from build123d import *

# Parameters (mm, degrees)
REVOLVE1_ANGLE           = 180
SKETCH3_R                = 2
BOSS_EXTRUDE1_DEPTH      = 13
BOSS_EXTRUDE8_REACH      = 185.507
BOSS_EXTRUDE8_END_RADIUS = 88.5
SKETCH7_R                = 10
SKETCH7_R_2              = 1.5
CUT_EXTRUDE1_DEPTH       = 10
BOSS_EXTRUDE11_DEPTH     = 25
FILLET1_R                = 20
CUT_EXTRUDE2_DEPTH       = 10
CUT_EXTRUDE3_DEPTH       = 10


with BuildPart() as part:
    # Sketch1 → Revolve1 (revolve)
    with BuildSketch(Plane(origin=(0, 0, 0), x_dir=(1, 0, 0), z_dir=(0, 1, 0))):
        Polygon((0, 75), (95, 75), (95, -95), (0, -125), align=None)
    revolve(axis=Axis((0, 0, 125), (0, 0, -1)), revolution_arc=REVOLVE1_ANGLE)

    # Sketch2 → Cut-Revolve3 (revolve, cut)
    with BuildSketch(Plane(origin=(0, 0, 0), x_dir=(1, 0, 0), z_dir=(0, 1, 0))):
        Polygon((0, 68.5), (0, -118.183600921), (88.5, -90.2362325), (88.5, 68.5), align=None)
    revolve(axis=Axis((0, 0, -68.5), (0, 0, 1)), mode=Mode.SUBTRACT)

    # Sketch3 → Boss-Extrude1 (add)
    with BuildSketch(Plane(origin=(0, 0, 0), x_dir=(1, 0, 0), z_dir=(0, 1, 0))):
        with Locations((-91.75, 56.5)):
            Circle(SKETCH3_R)
        with Locations((-91.75, 26.5)):
            Circle(SKETCH3_R)
        with Locations((-91.75, -18.5)):
            Circle(SKETCH3_R)
        with Locations((-91.75, -54.5)):
            Circle(SKETCH3_R)
        with Locations((91.75, -54.5)):
            Circle(SKETCH3_R)
        with Locations((91.75, -18.5)):
            Circle(SKETCH3_R)
        with Locations((91.75, 26.5)):
            Circle(SKETCH3_R)
        with Locations((91.75, 56.5)):
            Circle(SKETCH3_R)
    extrude(amount=BOSS_EXTRUDE1_DEPTH)

    # Boss-Extrude8: up to this cylinder (the profile starts inside it)
    boss_extrude8_end = Plane(origin=(0, 0, -64.648778), z_dir=(0, 0, -1)) * Cylinder(BOSS_EXTRUDE8_END_RADIUS, 549.014, mode=Mode.PRIVATE)
    # Sketch5 → Boss-Extrude8 (add, up to the surface)
    with BuildSketch(Plane(origin=(0, 0, 0), x_dir=(1, 0, 0), z_dir=(0, 1, 0)), mode=Mode.PRIVATE) as boss_extrude8_sk1:
        with BuildLine():
            Line((23.5, 63.447630747), (23.5, 68.5))
            Line((23.5, 68.5), (26.5, 68.5))
            Line((26.5, 68.5), (26.5, 63.447630747))
            Line((26.5, 63.447630747), (27.4, 63.447630747))
            ThreePointArc((27.4, 63.447630747), (25, 61.047630747), (22.6, 63.447630747))
            Line((22.6, 63.447630747), (23.5, 63.447630747))
        make_face()
    boss_extrude8_tool1 = extrude(boss_extrude8_sk1.sketch, amount=-BOSS_EXTRUDE8_REACH, mode=Mode.PRIVATE) & boss_extrude8_end
    add(boss_extrude8_tool1.solids().sort_by_distance((25, 0, -64.648778))[0])
    # Sketch5 → Boss-Extrude8 (add, up to the surface)
    with BuildSketch(Plane(origin=(0, 0, 0), x_dir=(1, 0, 0), z_dir=(0, 1, 0)), mode=Mode.PRIVATE) as boss_extrude8_sk2:
        with BuildLine():
            Line((-27.4, 63.447630747), (-26.5, 63.447630747))
            Line((-26.5, 63.447630747), (-26.5, 68.5))
            Line((-26.5, 68.5), (-23.5, 68.5))
            Line((-23.5, 68.5), (-23.5, 63.447630747))
            Line((-23.5, 63.447630747), (-22.6, 63.447630747))
            ThreePointArc((-22.6, 63.447630747), (-25, 61.047630747), (-27.4, 63.447630747))
        make_face()
    boss_extrude8_tool2 = extrude(boss_extrude8_sk2.sketch, amount=-BOSS_EXTRUDE8_REACH, mode=Mode.PRIVATE) & boss_extrude8_end
    add(boss_extrude8_tool2.solids().sort_by_distance((-25, 0, -64.648778))[0])

    # Sketch7 → Cut-Extrude1 (cut)
    with BuildSketch(Plane.XY.offset(-68.5)):
        Circle(SKETCH7_R)
        with Locations((20.425168298, -1.75)):
            Circle(SKETCH7_R_2)
        with Locations(Location((-20.425168298, -1.75, 0), (0, 0, 180))):
            Circle(SKETCH7_R_2)
    extrude(amount=-CUT_EXTRUDE1_DEPTH, mode=Mode.SUBTRACT)

    # Sketch8 → Boss-Extrude11 (add, symmetric)
    with BuildSketch(Plane.XY):
        Polygon((90.138781887, -30), (130.138781887, -30), (92.29707471, -22.5), align=None)
        Polygon((-130.138781887, -30), (-92.29707471, -22.5), (-90.138781887, -30), align=None)
    extrude(amount=BOSS_EXTRUDE11_DEPTH, both=True)

    # Fillet1
    fillet1_edges = [part.edges().sort_by_distance(p)[0] for p in [
        (0, -95, 95),
    ]]
    fillet(fillet1_edges, radius=FILLET1_R)

    # Sketch9 → Cut-Extrude2 (cut)
    with BuildSketch(Plane(origin=(-0.802339529, -4.048253002, 0), x_dir=(0.9809198737827295, -0.19441245129382567, 0), z_dir=(0.19441245129382567, 0.9809198737827295, 0))):
        with BuildLine():
            Line((114.199203035, -25), (133.488091041, -25))
            Line((133.488091041, -25), (133.488091041, 0))
            add(Edge.make_bspline(
                [(114.199203035, -25), (127.479134843, -22.055909998), (133.488091041, 0)],
                knots=[0, 0, 0, 1, 1, 1], degree=2))
        make_face()
    extrude(amount=-CUT_EXTRUDE2_DEPTH, mode=Mode.SUBTRACT)

    # Sketch10 → Cut-Extrude3 (cut)
    with BuildSketch(Plane(origin=(0.802339529, -4.048253002, 0), x_dir=(0.9809198737827294, 0.1944124512938259, 0), z_dir=(-0.1944124512938259, 0.9809198737827294, 0))):
        with BuildLine():
            Line((-114.199203035, -25), (-133.488091041, -25))
            Line((-133.488091041, -25), (-133.488091041, 0))
            add(Edge.make_bspline(
                [(-114.199203035, -25), (-129.601076996, -21.529037797), (-133.488091041, 0)],
                knots=[0, 0, 0, 1, 1, 1], degree=2))
        make_face()
    extrude(amount=-CUT_EXTRUDE3_DEPTH, mode=Mode.SUBTRACT)


solid = part.part
CAD build for the part. Positions are in the model's coordinates, mm. A direction names the side the tool comes from. Coordinates: 2 decimals unless noted, no trailing zeros. Order: outer loops, then holes, each group sorted by start corner. A loop starts at its lowest first (then second) coordinate and runs counter-clockwise, first axis right, second up. Notation, with made-up numbers: (33.5, 80.25) -> (62.5, 80.25) arc R10 cw to (62.5, 96.25) -> close; hole circle Ø10 at (39.25, 22). An arc over 180 degrees is marked (long way). Answer in a Markdown table with one row per item.
1) Drill centre lines: line 1 (X direction, y = -1, z = -71); line 2 (X direction, y = -35, z = 84.5) (3 decimals); line 3 (Z direction, x = 28, y = -67.5). Where is each one in solid material? Low to high.
Check values:
| item | result |
|---|---|
| line 1 | -94.99 to -21.72, -19.13 to -9.95, 9.95 to 19.13, 21.72 to 94.99 |
| line 2 | -87.847 to -81.285, 81.285 to 87.847 |
| line 3 | -75 to -68.5, 95.11 to 101.92 |
2) Band-saw the part on A-A (y = 6.5). List the corners of the cut face in (x, z).
Check values:
| item | result |
|---|---|
| outline | circle Ø4 at (-91.75, -56.5); circle Ø4 at (-91.75, -26.5); circle Ø4 at (-91.75, 18.5); circle Ø4 at (-91.75, 54.5); circle Ø4 at (91.75, -56.5); circle Ø4 at (91.75, -26.5); circle Ø4 at (91.75, 18.5); circle Ø4 at (91.75, 54.5) |
3) Band-saw the part on C-C (z = 36). List the corners of the cut face in (x, y), and give its area (3 significant figures).
Check values:
| item | result |
|---|---|
| outline | (-95, 0) arc R95 ccw to (95, 0) -> (88.5, 0) arc R88.5 cw to (-88.5, 0) -> close |
| area | 1,870 mm2 |
4) Flat gauge pins, fed straight in: P1, Ø12, axis at y = -79, z = 74, coming from the +X side; P2, Ø12, axis at x = -46.5, z = -31.5, coming from the +Y side; P3, Ø2.5, axis at x = 103.5, y = -28, coming from the +Z side. Where does each tip first touch, or does it go through?
Check values:
| item | result |
|---|---|
| P1 | x = 60.79 |
| P2 | y = -71.25 |
| P3 | z = 25 |
5) Band-saw the part on B-B (z = -6.5). List the corners of the cut face in (x, y).
Check values:
| item | result |
|---|---|
| outline | (-130.14, -30) -> (-90.14, -30) arc R95 ccw to (90.14, -30) -> (130.14, -30) -> (92.3, -22.5) arc R95 ccw to (95, 0) -> (88.5, 0) arc R88.5 cw to (-88.5, 0) -> (-95, 0) arc R95 ccw to (-92.3, -22.5) -> close |
6) Which spindle directions (+Z, -Z, +X, -X, +Y, -Y) get a long thin tool onto all of the face, cutting with end or side? Do faces 1 (the face through (50, -32, -68.5)), 2 (the face through (0, -10, -72)), 3 (the face through (-105, -27, -25)). Say none if no direction does.
Check values:
| item | result |
|---|---|
| face 1 | +Y |
| face 2 | -Z, +Y |
| face 3 | -Z, -X, -Y |
